Can you work these out from the model? Positions are in its coordinate system, mm. Face numbers are marked on the shaded views. A direction names the side the tool comes from. Give positions to 0.01 mm unless a question says otherwise; leave off trailing zeros. Order: outer loops, then holes, each group sorted by start corner. A loop starts at its lowest first (then second) coordinate and runs counter-clockwise, first axis right, second up. Notation, with made-up numbers: (-33, 38) - (-20, 38) arc R18 cw to (-20, 44) - close; hole circle Ø2 at (55.25, 32). An arc over 180 degrees is marked (long way). Use one line per item in the form item = value. Start each with the question number.
1) Suppose I cut it at C-C, the plane z = 2.25. Write out the boundary of the cut face in (x, y) (3 decimals).
2) Suppose I cut it at D-D, the plane x = 0. Write out the boundary of the cut face in (y, z) (3 decimals), and give its area (3 significant figures).
3) We'd pull the mould along Y, two halves only. Please class the marked faces 4, 5 and 6: released by +Y, released by -Y, zero draft, split by the parting line, or undercut.
4) Suppose I cut it at A-A, the plane y = 0. Write out the boundary of the cut face in (x, z) (3 decimals), and give its area (3 significant figures).
5) For pin 1 (1.6 mm diameter, centred on x = 16.5, z = 1, fed in from +Y); pin 2 (1.5 mm diameter, centred on y = -2, z = 1, fed in from +X), each with a flat end and sliding along its axis, tell me the tip position at first contact or that it passes through.
6) Please list where these lines run through material, in increasing order: probe 1 along X at (y, z) = (0, 1.05) (3 decimals); probe 2 along Y at (x, z) = (16, 2.95); probe 3 along Y at (x, z) = (-13, 0.75).
7) Which directions (+Z, -Z, +X, -X, +Y, -Y) give clear straight access to the entire face, cutting with the end or side of a thin tool? Please do the marked faces 1, 2 and 3.
8) Suppose I cut it at B-B, the plane x = -5.5. Write out the boundary of the cut face in (y, z) (3 decimals), and give its area (3 significant figures).
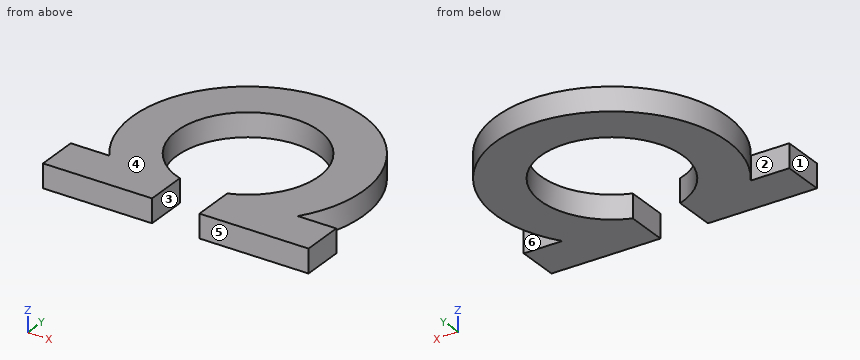
```python
from build123d import *

# Parameters (mm, degrees)
PAD_DEPTH = 3.175


with BuildPart() as part:
    # Sketch → Pad (new body)
    with BuildSketch(Plane.XY):
        with BuildLine():
            Line((-17.78, -8.980256), (-17.78, -14.568256))
            Line((-17.78, -14.568256), (-3.175, -14.568256))
            Line((-3.175, -14.568256), (-3.175, -8.980256))
            ThreePointArc((3.175, -8.980256), (0, 9.525), (-3.175, -8.980256))
            Line((3.175, -8.980256), (3.175, -14.568256))
            Line((3.175, -14.568256), (17.78, -14.568256))
            Line((17.78, -14.568256), (17.78, -8.980256))
            Line((17.78, -8.980256), (12.626125, -8.980256))
            ThreePointArc((12.626125, -8.980256), (0, 15.494), (-12.626125, -8.980256))
            Line((-17.78, -8.980256), (-12.626125, -8.980256))
        make_face()
    extrude(amount=PAD_DEPTH)


solid = part.part
```
Result sheet:
q1.outline = (-17.78, -14.568) - (-3.175, -14.568) - (-3.175, -8.98) arc R9.525 cw (long way) to (3.175, -8.98) - (3.175, -14.568) - (17.78, -14.568) - (17.78, -8.98) - (12.626, -8.98) arc R15.494 ccw (long way) to (-12.626, -8.98) - (-17.78, -8.98) - close
q2.outline = (9.525, 0) - (15.494, 0) - (15.494, 3.175) - (9.525, 3.175) - close
q2.area = 19.0 mm²
q3.face_4 = zero draft
q3.face_5 = released by -Y
q3.face_6 = undercut
q4.outline = (-15.494, 0) - (-9.525, 0) - (-9.525, 3.175) - (-15.494, 3.175) - close; (9.525, 0) - (15.494, 0) - (15.494, 3.175) - (9.525, 3.175) - close
q4.area = 37.9 mm²
q5.pin_1 = -8.98
q5.pin_2 = 15.44
q6.probe_1 = -15.494 to -9.525, 9.525 to 15.494
q6.probe_2 = -14.57 to -8.98
q6.probe_3 = -14.57 to -8.98, -8.43 to 8.43
q7.face_1 = +Z, -Z, -X, +Y, -Y
q7.face_2 = +Z, -Z, -X
q7.face_3 = +Z, -Z, -Y
q8.outline = (-14.568, 0) - (-7.777, 0) - (-7.777, 3.175) - (-14.568, 3.175) - close; (7.777, 0) - (14.485, 0) - (14.485, 3.175) - (7.777, 3.175) - close
q8.area = 42.9 mm²
